```python
from build123d import *

# Parameters (mm, degrees)
SKETCH1_W           = 72
SKETCH1_H           = 67
BOSS_EXTRUDE1_DEPTH = 6
SKETCH2_R           = 5
SKETCH2_R_2         = 2
CUT_EXTRUDE1_DEPTH  = 6
SKETCH3_R           = 7.5
CUT_EXTRUDE2_DEPTH  = 4.2
SKETCH5_R           = 2
CUT_EXTRUDE3_DEPTH  = 10
SKETCH6_R           = 1.5
CUT_EXTRUDE4_DEPTH  = 10


with BuildPart() as part:
    # Sketch1 → Boss-Extrude1 (new body)
    with BuildSketch(Plane(origin=(0, 0, 0), x_dir=(1, 0, 0), z_dir=(0, 1, 0))):
        Rectangle(SKETCH1_W, SKETCH1_H)
    extrude(amount=BOSS_EXTRUDE1_DEPTH)

    # Sketch2 → Cut-Extrude1 (cut)
    with BuildSketch(Plane(origin=(0, 6, 0), x_dir=(1, 0, 0), z_dir=(0, 1, 0))):
        with Locations(Location((0, 0, 0), (0, 0, 270))):
            Circle(SKETCH2_R)
        with Locations(Location((-6.5, 15.5, 0), (0, 0, 270))):
            Circle(SKETCH2_R_2)
        with Locations(Location((-6.5, -15.5, 0), (0, 0, 270))):
            Circle(SKETCH2_R_2)
    extrude(amount=-CUT_EXTRUDE1_DEPTH, mode=Mode.SUBTRACT)

    # Sketch3 → Cut-Extrude2 (cut)
    with BuildSketch(Plane(origin=(0, 6, 0), x_dir=(1, 0, 0), z_dir=(0, 1, 0))):
        with Locations(Location((0, 0, 0), (0, 0, 270))):
            Circle(SKETCH3_R)
    extrude(amount=-CUT_EXTRUDE2_DEPTH, mode=Mode.SUBTRACT)

    # Sketch5 → Cut-Extrude3 (cut)
    with BuildSketch(Plane(origin=(0, 6, 0), x_dir=(1, 0, 0), z_dir=(0, 1, 0))):
        with Locations(Location((12, 0, 0), (0, 0, 270))):
            Circle(SKETCH5_R)
    extrude(amount=-CUT_EXTRUDE3_DEPTH, mode=Mode.SUBTRACT)

    # Sketch6 → Cut-Extrude4 (cut)
    with BuildSketch(Plane.XZ):
        with Locations(Location((-25, 24.5, 0), (0, 0, 270))):
            Circle(SKETCH6_R)
        with Locations(Location((25, 24.5, 0), (0, 0, 90))):
            Circle(SKETCH6_R)
        with Locations(Location((-33, 15, 0), (0, 0, 270))):
            Circle(SKETCH6_R)
        with Locations(Location((33, 15, 0), (0, 0, 90))):
            Circle(SKETCH6_R)
        with Locations(Location((33, -15, 0), (0, 0, 270))):
            Circle(SKETCH6_R)
        with Locations(Location((-33, -15, 0), (0, 0, 90))):
            Circle(SKETCH6_R)
        with Locations(Location((25, -24.5, 0), (0, 0, 270))):
            Circle(SKETCH6_R)
        with Locations(Location((-25, -24.5, 0), (0, 0, 90))):
            Circle(SKETCH6_R)
    extrude(amount=-CUT_EXTRUDE4_DEPTH, mode=Mode.SUBTRACT)


solid = part.part
```
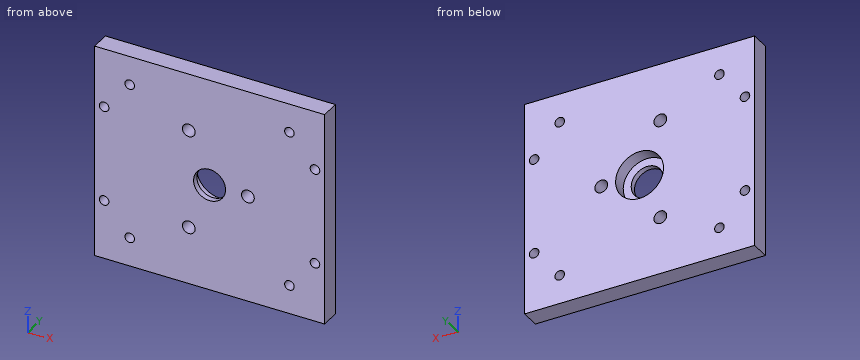
Part model, mm, in its own coordinate system. Give positions to 0.01 mm unless a question says otherwise; leave off trailing zeros. Write each loop counter-clockwise with the first axis right and the second up, starting at its lowest first coordinate (ties: lowest second). Pieces come first, ordered by that corner, then holes. Notation, with made-up numbers: M 45.25,19 L 82.25,19 A24 cw 82.25,57 Z; hole C 76,16.5 d8. An arc over 180 degrees is marked long. Use CSV: the item, a comma, the result in double quotes.
Item 1: Slice it at A-A on z = -24.5. Write the cut outline in (x, y), plus the area to 3 significant figures.
Taken from the geometry:
outline,"M -36,0 L -26.5,0 L -26.5,6 L -36,6 Z; M -23.5,0 L 23.5,0 L 23.5,6 L -23.5,6 Z; M 26.5,0 L 36,0 L 36,6 L 26.5,6 Z"
area,"396 mm²"
Item 2: Slice it at C-C on y = 4.35. State how many separate pieces and enclosed holes the cut face has, plus the area to 3 significant figures.
Taken from the geometry:
separate pieces,"1"
enclosed holes,"12"
area,"4,550 mm²"
Item 3: Slice it at D-D on x = 33. Write the cut outline in (y, z).
Taken from the geometry:
outline,"M 0,-33.5 L 6,-33.5 L 6,-16.5 L 0,-16.5 Z; M 0,-13.5 L 6,-13.5 L 6,13.5 L 0,13.5 Z; M 0,16.5 L 6,16.5 L 6,33.5 L 0,33.5 Z"
Item 4: Slice it at B-B on x = 0. Write the cut outline in (y, z), plus the area to 3 significant figures.
Taken from the geometry:
outline,"M 0,-33.5 L 6,-33.5 L 6,-7.5 L 1.8,-7.5 L 1.8,-5 L 0,-5 Z; M 0,5 L 1.8,5 L 1.8,7.5 L 6,7.5 L 6,33.5 L 0,33.5 Z"
area,"321 mm²"
Item 5: Drill centre lines: probe 1 along X at (y, z) = (3.5, -24.5); probe 2 along X at (y, z) = (5.1, 0); probe 3 along X at (y, z) = (3.15, -15). Where is each one in solid material? Low to high.
Taken from the geometry:
probe 1,"x = -36 to -26.5, -23.5 to 23.5, 26.5 to 36"
probe 2,"x = -36 to -7.5, 7.5 to 10, 14 to 36"
probe 3,"x = -36 to -34.5, -31.5 to -8.44, -4.56 to 31.5, 34.5 to 36"
